from build123d import *

# Parameters (mm, degrees)
SKETCH1_W                       = 30
SKETCH1_H                       = 50
BOSS_EXTRUDE1_DEPTH             = 5
M4X0_7_TAPPED_HOLE1_D           = 3.3
M4X0_7_TAPPED_HOLE1_CSINK_D     = 4.05
M4X0_7_TAPPED_HOLE1_CSINK_ANGLE = 100
CHAMFER1_SIZE                   = 3


with BuildPart() as part:
    # Sketch1 → Boss-Extrude1 (new body)
    with BuildSketch(Plane(origin=(0, 0, 0), x_dir=(1, 0, 0), z_dir=(0, 1, 0))):
        Rectangle(SKETCH1_W, SKETCH1_H)
    extrude(amount=BOSS_EXTRUDE1_DEPTH)

    # M4x0.7 Tapped Hole1 (through all)
    with Locations(Plane(origin=(0, 5, 0), x_dir=(1, 0, 0), z_dir=(0, 1, 0))):
        with Locations((-5.5, -15), (-5.5, 0), (4.5, 0), (4.5, 15)):
            CounterSinkHole(M4X0_7_TAPPED_HOLE1_D / 2, M4X0_7_TAPPED_HOLE1_CSINK_D / 2, counter_sink_angle=M4X0_7_TAPPED_HOLE1_CSINK_ANGLE)

    # Chamfer1
    chamfer1_edges = [part.edges().sort_by_distance(p)[0] for p in [
        (15, 2.5, 25),
        (-15, 2.5, 25),
        (-15, 2.5, -25),
        (15, 2.5, -25),
    ]]
    chamfer(chamfer1_edges, length=CHAMFER1_SIZE)


solid = part.part
Design review of the part built by this model. Coordinates are the model's own, in mm. Round coordinates to 2 decimals unless told otherwise and drop trailing zeros. Loops run counter-clockwise (first coordinate to the right, second up) from the corner with the lowest first, then second, coordinate; pieces in that order, holes last. Notation, with made-up numbers: (-9.75, -18) - (18.25, -18) arc R20 ccw to (18.25, -8) - close; hole circle Ø9 at (-29.75, -32.75). An arc over 180 degrees is marked (long way). One line per item, written item: value. Start each with the question number.
1) Consider section D-D on y = 3.1. Give the boundary of the cut face in (x, z), then the cut area to 3 significant figures.
2) Consider section C-C on z = 15. Give the boundary of the cut face in (x, y) (3 decimals), then the cut area to 3 significant figures.
3) Consider section B-B on x = 4.5. Give the boundary of the cut face in (y, z) (3 decimals), then the cut area to 3 significant figures.
4) Consider section A-A on z = 0. Give the boundary of the cut face in (x, y) (3 decimals).
5) To check wall thickness, follow L1, parallel to Z at x = 4.5, y = 1.1; L2, parallel to Z at x = -5.5, y = 1.3; L3, parallel to X at y = 0.6, z = -1. State the ranges of each line that lie inside material, in increasing order. Write a range as from..to.
6) Draft analysis for pull direction X (two halves, no side actions). For faces 1 (the flat face through (-15, 2, 0)), 2 (the flat face through (0, 2, 25)), 3 (the cylindrical face through (-3.85, 2.31, -0.07)), state which applies: +X half, -X half, draft (parallel to the pull), parting line (faces both ways), or undercut.
Reported:
1. outline: (-15, -22) - (-12, -25) - (12, -25) - (15, -22) - (15, 22) - (12, 25) - (-12, 25) - (-15, 22) - close; hole circle Ø3.3 at (-5.5, 0); hole circle Ø3.3 at (-5.5, 15); hole circle Ø3.3 at (4.5, -15); hole circle Ø3.3 at (4.5, 0)
1. area: 1,450 mm^2
2. outline: (-15, 0) - (-7.15, 0) - (-7.15, 4.685) - (-7.525, 5) - (-15, 5) - close; (-3.85, 0) - (15, 0) - (15, 5) - (-3.475, 5) - (-3.85, 4.685) - close
2. area: 133 mm^2
3. outline: (0, -25) - (5, -25) - (5, -17.025) - (4.685, -16.65) - (0, -16.65) - close; (0, -13.35) - (4.685, -13.35) - (5, -12.975) - (5, -2.025) - (4.685, -1.65) - (0, -1.65) - close; (0, 1.65) - (4.685, 1.65) - (5, 2.025) - (5, 25) - (0, 25) - close
3. area: 217 mm^2
4. outline: (-15, 0) - (-7.15, 0) - (-7.15, 4.685) - (-7.525, 5) - (-15, 5) - close; (-3.85, 0) - (2.85, 0) - (2.85, 4.685) - (2.475, 5) - (-3.475, 5) - (-3.85, 4.685) - close; (6.15, 0) - (15, 0) - (15, 5) - (6.525, 5) - (6.15, 4.685) - close
5. L1: z = -25..-16.65, -13.35..-1.65, 1.65..25
5. L2: z = -25..-1.65, 1.65..13.35, 16.65..25
5. L3: x = -15..-6.81, -4.19..3.19, 5.81..15
6. face 1: -X half
6. face 2: draft
6. face 3: undercut
